Geometry: final body of the model. Coordinates: model frame, mm. A direction names the side the tool comes from. Coordinates: 2 decimals unless noted, no trailing zeros. Loops run counter-clockwise (first coordinate to the right, second up) from the corner with the lowest first, then second, coordinate; pieces in that order, holes last. Notation, with made-up numbers: (34.5, -21) - (85.5, -21) arc R23 ccw to (85.5, -2) - close; hole circle Ø7 at (9, -17.75). An arc over 180 degrees is marked (long way). Answer in a Markdown table with one row per item.
from build123d import *

# Parameters (mm, degrees)
SKETCH1_R                = 2.5
SKETCH1_R_2              = 2.035533906
SKETCH1_R_3              = 1.5
BOSS_EXTRUDE1_DEPTH      = 6
SKETCH1_3_R              = 2.5
SKETCH1_3_R_2            = 2.035533906
CUT_EXTRUDE1_DEPTH       = 1
SKETCH2_R                = 1.5
SKETCH2_R_2              = 1
BOSS_EXTRUDE3_DEPTH      = 1
BOSS_EXTRUDE3_DEPTH_BACK = 1


with BuildPart() as part:
    # Sketch1 → Boss-Extrude1 (new body)
    with BuildSketch(Plane(origin=(0, 0, 0), x_dir=(1, 0, 0), z_dir=(0, 1, 0))):
        Circle(SKETCH1_R)
        Circle(SKETCH1_R_2, mode=Mode.SUBTRACT)
        Circle(SKETCH1_R_2)
        Circle(SKETCH1_R_3, mode=Mode.SUBTRACT)
    extrude(amount=BOSS_EXTRUDE1_DEPTH)

    # Sketch1_3 → Cut-Extrude1 (cut)
    with BuildSketch(Plane(origin=(0, 0, 0), x_dir=(1, 0, 0), z_dir=(0, 1, 0))):
        Circle(SKETCH1_3_R)
        Circle(SKETCH1_3_R_2, mode=Mode.SUBTRACT)
    extrude(amount=CUT_EXTRUDE1_DEPTH, mode=Mode.SUBTRACT)

    # Sketch2 → Boss-Extrude3 (add, two sides)
    with BuildSketch(Plane(origin=(0, 6, 0), x_dir=(1, 0, 0), z_dir=(0, 1, 0))) as boss_extrude3_sk:
        Circle(SKETCH2_R)
        Circle(SKETCH2_R_2, mode=Mode.SUBTRACT)
    extrude(amount=BOSS_EXTRUDE3_DEPTH)
    extrude(boss_extrude3_sk.sketch, amount=-BOSS_EXTRUDE3_DEPTH_BACK)


solid = part.part
(1) Access query for faces 1 (the face through (0, 6, 2)), 2 (the face through (-0.54, 3.46, 2.44)), 3 (the face through (-0.26, 0.49, -2.02)). Directions: +Z, -Z, +X, -X, +Y, -Y. A direction counts if a zero-diameter tool reaches every point of the face in a straight line with its end or side. Return the directions, or none.
Verdict:
| item | result |
|---|---|
| face 1 | +Y |
| face 2 | +Y, -Y |
| face 3 | -Y |
(2) Cut plane D-D on x = 1.25. Output: boundary loops of the cut face in (y, z).
Verdict:
| item | result |
|---|---|
| outline | (0, -1.61) - (1, -1.61) - (1, -2.17) - (6, -2.17) - (6, -0.83) - (7, -0.83) - (7, 0.83) - (6, 0.83) - (6, 2.17) - (1, 2.17) - (1, 1.61) - (0, 1.61) - (0, 0.83) - (5, 0.83) - (5, -0.83) - (0, -0.83) - close |
(3) Cut plane C-C on y = 5.75. Output: boundary loops of the cut face in (x, z), then the cut area to 3 significant figures.
Verdict:
| item | result |
|---|---|
| outline | circle Ø5 at (0, 0); hole circle Ø2 at (0, 0) |
| area | 16.5 mm² |
(4) Pull-direction query (X, two-part tool) for faces 4 (the face through (-1, 1, 2)), 5 (the face through (-1.5, 2.46, -0.07)), 6 (the face through (-1.5, 6.49, -0.07)); classes: pulls with the +X half, pulls with the -X half, needs draft (parallel to the pull), parting line crosses it, or undercut.
Verdict:
| item | result |
|---|---|
| face 4 | needs draft |
| face 5 | undercut |
| face 6 | parting line crosses it |
(5) Cut plane A-A on x = 0. Output: boundary loops of the cut face in (y, z).
Verdict:
| item | result |
|---|---|
| outline | (0, -2.04) - (1, -2.04) - (1, -2.5) - (6, -2.5) - (6, -1.5) - (7, -1.5) - (7, -1) - (5, -1) - (5, -1.5) - (0, -1.5) - close; (0, 1.5) - (5, 1.5) - (5, 1) - (7, 1) - (7, 1.5) - (6, 1.5) - (6, 2.5) - (1, 2.5) - (1, 2.04) - (0, 2.04) - close |
(6) Cut plane B-B on z = 0. Output: boundary loops of the cut face in (x, y), then the cut area to 3 significant figures.
Verdict:
| item | result |
|---|---|
| outline | (-2.5, 1) - (-2.04, 1) - (-2.04, 0) - (-1.5, 0) - (-1.5, 5) - (-1, 5) - (-1, 7) - (-1.5, 7) - (-1.5, 6) - (-2.5, 6) - close; (1, 5) - (1.5, 5) - (1.5, 0) - (2.04, 0) - (2.04, 1) - (2.5, 1) - (2.5, 6) - (1.5, 6) - (1.5, 7) - (1, 7) - close |
| area | 13.1 mm² |
(7) Ray query, probe 1 along Z at (x, y) = (0, 5.5); probe 2 along Z at (x, y) = (0, 1.75); probe 3 along X at (y, z) = (6.6, 0). Return the intervals inside material, ascending.
Verdict:
| item | result |
|---|---|
| probe 1 | z = -2.5 to -1, 1 to 2.5 |
| probe 2 | z = -2.5 to -1.5, 1.5 to 2.5 |
| probe 3 | x = -1.5 to -1, 1 to 1.5 |
(8) First-contact query: pin 1 Ø1.5 at (x, y) = (-1.5, 1.5) entering from -Z; pin 2 Ø2.5 at (x, z) = (0, 0) entering from -Y. Flat tips, straight axial feed; report the tip coordinate or a pass-through.
Verdict:
| item | result |
|---|---|
| pin 1 | stops at z = -2.38 |
| pin 2 | stops at y = 5 |
